Input: part model. Units: mm. Frame: model coordinates. Face numbers are marked on the shaded views. A direction names the side the tool comes from. Round coordinates to 2 decimals unless told otherwise and drop trailing zeros. Order: outer loops, then holes, each group sorted by start corner. A loop starts at its lowest first (then second) coordinate and runs counter-clockwise, first axis right, second up. Notation, with made-up numbers: M 5,-6 L 50,-6 A5 cw 50,2 Z; hole C 1,52 d2. An arc over 180 degrees is marked long. One line per question, with ' | ' between items.
Autodesk Inventor part; units mm, degrees
ref_plane "YZ Plane" through (0, 0, 0) normal (1, 0, 0) x (0, 1, 0)
ref_plane "XZ Plane" through (0, 0, 0) normal (0, 1, 0) x (-1, 0, 0)
ref_plane "XY Plane" through (0, 0, 0) normal (0, 0, 1) x (1, 0, 0)
sketch "Эскиз1" plane through (0, 0, 0) normal (0, 1, 0) x (-1, 0, 0)
  line L0 (54, 15) -> (-54, 15)
  line L1 (-54, 15) -> (-54, -15)
  line L2 (-54, -15) -> (54, -15)
  line L3 (54, -15) -> (54, 15)
  line L4 (-54, 15) -> (54, -15) construction
  line L5 (-54, -15) -> (54, 15) construction
  line L6 (0, -21) -> (0, 21) construction
  line L7 (44, -13) -> (7.0585, -13)
  line L8 (-44, -13) -> (-44, 13)
  line L9 (-44, 13) -> (0, 13)
  line L10 (44, 13) -> (44, 2.0855)
  line L11 (75.6, 0) -> (-75.6, 0) construction
  line L12 (49, -15) -> (49, 15) construction
  line L13 (0, -13) -> (44, 0)
  line L14 (44, -2.0855) -> (7.0585, -13)
  line L15 (0, -15) -> (0, -13) construction
  line L16 (0, 13) -> (0, 15) construction
  line L17 (44, -2.0855) -> (43.4333, -0.1674) construction
  line L18 (44, 0) -> (0, 13)
  line L19 (44, 2.0855) -> (7.0585, 13)
  line L20 (44, 2.0855) -> (43.4333, 0.1674) construction
  line L21 (44, 2.0855) -> (44, -2.0855) construction
  line L22 (44, -2.0855) -> (44, -13)
  line L23 (7.0585, -13) -> (0, -13) construction
  line L24 (0, -13) -> (-44, -13)
  line L25 (7.0585, 13) -> (44, 13)
  line L26 (0, 13) -> (7.0585, 13) construction
  point P0 (0, 0)
  point P1 (0, -14)
  point P2 (0, 14)
  point P3 (0, 0)
  dimension "d0" = 108
  dimension "d8" = 10
  dimension "d9" = 5
  dimension "d28" = 26
  dimension "d46" = 2
  dimension "d47" = 10
extrude "Выдавливание1" add sketch "Эскиз1" along normal blind 2
sketch "Эскиз2" plane through (0, 0, 0) normal (0, 1, 0) x (-1, 0, 0)
  line L0 (-42, -13) -> (-42, 13) construction
  line L1 (-42, -13) -> (-29, -13) construction
  line L2 (-10.5, -13) -> (-10.5, -15)
  line L3 (-10.5, -15) -> (-44, -15)
  line L4 (-42, 13) -> (-29, 13) construction
  line L5 (-10.5, 15) -> (-44, 15)
  line L6 (-10.5, 13) -> (-10.5, 15)
  arc A0 (-29, 13) -> (-29, -13) centre (-29, 0) ccw
  line L7 (-29, -13) -> (-10.5, -13)
  line L8 (-29, 13) -> (-10.5, 13)
  line L9 (-44, -15) -> (-44, 15)
  line L10 (-44, -13) -> (-44, 13) construction
  line L11 (0, -13) -> (-44, -13) construction
  line L12 (-54, -15) -> (54, -15) construction
  line L13 (-44, 13) -> (0, 13) construction
  line L14 (54, 15) -> (-54, 15) construction
  point P0 (0, 0)
  dimension "d17" = 31.5
  dimension "d48" = 2
extrude "Выдавливание2" add sketch "Эскиз2" along normal blind 13
sketch "Эскиз4" plane through (0, 2, 0) normal (0, 1, 0) x (1, 0, 0)
  line L0 (-54, 15) -> (-54, -15) construction
  line L1 (-44, 13) -> (-54, 13)
  line L2 (-54, 13) -> (-54, 15)
  line L3 (-54, 15) -> (-44, 15)
  line L4 (-44, 15) -> (-44, 13)
  line L5 (44, -13) -> (0, -13) construction
  line L6 (-54, -15) -> (54, -15) construction
  line L7 (-44, -13) -> (-54, -13)
  line L8 (-54, -13) -> (-54, -15)
  line L9 (-54, -15) -> (-44, -15)
  line L10 (-44, -15) -> (-44, -13)
  point P0 (0, 0)
  point P1 (10.5, -13)
  point P2 (-44, -15)
extrude "Выдавливание4" add sketch "Эскиз4" along normal blind 45
sketch "Эскиз3" plane through (-54, 0, 15) normal (0, 0, 1) x (1, 0, 0)
  line L0 (64.5, 2) -> (64.5, 13) construction
  line L1 (64.5, 13) -> (74.5, 13) construction
  line L2 (74.5, 13) -> (74.5, 3) construction
  line L3 (74.5, 3) -> (64.5, 3) construction
  line L4 (64.5, 3) -> (64.5, 13) construction
  line L5 (64.5, 2) -> (54, 2) construction
  line L6 (74.5, 3) -> (64.5, 13) construction
  line L7 (74.5, 13) -> (64.5, 3) construction
  circle A0 centre (69.5, 8) radius 0.5
  line L8 (0, 47) -> (10, 47) construction
  line L9 (10, 2) -> (10, 47) construction
  line L10 (0, 47) -> (10, 47) construction
  line L11 (10, 47) -> (10, 37) construction
  line L12 (10, 37) -> (0, 37) construction
  line L13 (0, 37) -> (0, 47) construction
  line L14 (0, 37) -> (10, 47) construction
  line L15 (0, 0) -> (0, 47) construction
  line L16 (10, 37) -> (0, 47) construction
  circle A1 centre (5, 42) radius 0.5
  point P0 (54, 0)
  point P1 (128, 2)
  dimension "d20" = 10
  dimension "d21" = 1
  dimension "d26" = 10
  dimension "d27" = 1
hole "Отверстие1" at (-49, 42, 15) at (15.5, 8, 15) direction (0, 0, -1) diameter 1 depth 2 countersink diameter 1.5 countersink angle 90
mirror "Зеркальное отражение1" about plane through (0, 0, 0) normal (0, 0, 1) of "Отверстие1"
sketch "Эскиз5" plane through (0, 2, 0) normal (0, 1, 0) x (1, 0, 0)
  line L0 (10.5, 13) -> (10.5, 15) construction
  line L1 (-44, 15) -> (10.5, 15) construction
  line L2 (-54, 15) -> (-44, 15) construction
  line L3 (-54, 13) -> (-54, 15) construction
  line L4 (-44, 13) -> (-54, 13) construction
  line L5 (-44, -13) -> (-44, -15) construction
  line L6 (-44, -15) -> (-54, -15) construction
  line L7 (-54, -15) -> (-54, -13) construction
  line L8 (-54, -13) -> (-54, 13) construction
  line L9 (10.5, -15) -> (10.5, -13) construction
  line L10 (10.5, 15) -> (44, 15) construction
  line L11 (54, -15) -> (44, -15) construction
  line L12 (54, 15) -> (54, -15) construction
  line L13 (44, 15) -> (54, 15) construction
  line L14 (-44, 15) -> (-44, 13) construction
  line L15 (-54, -13) -> (-44, -13) construction
  line L16 (44, -15) -> (10.5, -15) construction
  line L17 (54, 15) -> (-54, 15) construction
  line L18 (54, 15) -> (44, 0) construction
  line L19 (-54, -15) -> (54, -15) construction
  line L20 (54, -15) -> (44, 0) construction
  line L21 (-54, 13) -> (-44, -13) construction
  line L22 (-44, -13) -> (-44, -2.0855) construction
  line L23 (-54, -13) -> (-44, 13) construction
  line L24 (54, -15) -> (54, 15) construction
  line L25 (54, 0) -> (44, 15) construction
  line L26 (44, -15) -> (54, 0) construction
  circle A0 centre (-49, 0) radius 0.5
  circle A1 centre (49, 7.5) radius 0.5
  circle A2 centre (49, -7.5) radius 0.5
  line L27 (-44, 2.0855) -> (-7.0585, 13)
  line L28 (-7.0585, 13) -> (-44, 13)
  line L29 (-44, -13) -> (-7.0585, -13)
  line L30 (-7.0585, -13) -> (-44, -2.0855)
  line L31 (-44, -2.0855) -> (-44, -13)
  line L32 (-44, 13) -> (-44, 2.0855)
  line L33 (10.5, 13) -> (0, 13)
  line L34 (0, 13) -> (-44, 0)
  line L35 (-44, 0) -> (0, -13)
  line L36 (0, -13) -> (10.5, -13)
  line L37 (10.5, -13) -> (29, -13)
  arc A3 (29, -13) -> (29, 13) centre (29, 0) ccw
  line L38 (29, 13) -> (10.5, 13)
  line L39 (44, 15) -> (44, -15)
  line L40 (10.5, -15) -> (-44, -15)
  point P0 (0, 0)
  dimension "d38" = 1
hole "Отверстие2" at (-49, 2, 0) at (49, 2, 7.5) at (49, 2, -7.5) direction (0, -1, 0) diameter 1 end through all countersink diameter 1.5 countersink angle 90
properties part number "frame"
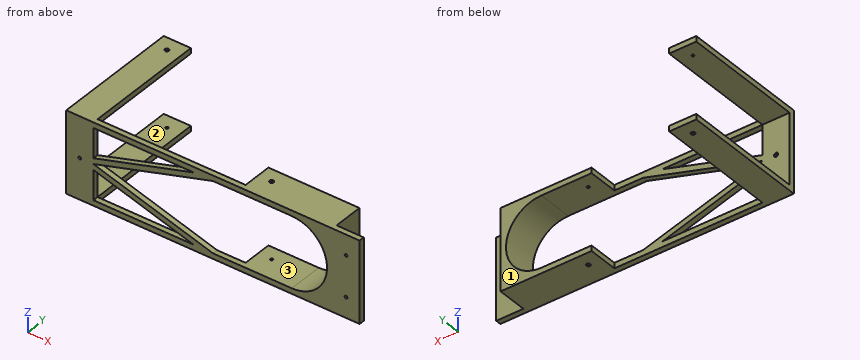
Item 1: Section query A-A, the plane y = 5.5. Return loops of the section in (x, z).
Report:
outline: M -54,-15 L -44,-15 L -44,-13 L -54,-13 Z; M -54,13 L -44,13 L -44,15 L -54,15 Z; M 10.5,-15 L 44,-15 L 44,15 L 10.5,15 L 10.5,13 L 29,13 A13 cw 29,-13 L 10.5,-13 Z
Item 2: Section query C-C, the plane y = 21.5. Return loops of the section in (x, z).
Report:
outline: M -54,-15 L -44,-15 L -44,-13 L -54,-13 Z; M -54,13 L -44,13 L -44,15 L -54,15 Z
Item 3: First-contact query: pin 1 (1 mm diameter, centred on y = 16, z = -14, fed in from +X); pin 2 (5 mm diameter, centred on y = 10, z = 0, fed in from +X); pin 3 (10 mm diameter, centred on x = -6.5, z = 6.5, fed in from +Y). Flat tips, straight axial feed; report the tip coordinate or a pass-through.
Report:
pin 1: x = -44 | pin 2: x = 44 | pin 3: y = 2
Item 4: Section query B-B, the plane x = 26.5. Return loops of the section in (y, z).
Report:
outline: M 0,-15 L 13,-15 L 13,-13 L 0,-13 Z; M 0,13 L 13,13 L 13,15 L 0,15 Z
Item 5: Line query: line 1 along X through (y, z) = (8, 14); line 2 along Y through (x, z) = (-49, -14.25); line 3 along Y through (x, z) = (15.5, 13.6). Output: solid intervals per line, ascending. Write a range as from..to.
Report:
line 1: -54..-44, 10.5..15, 16..44 | line 2: 0..41.5, 42.5..47 | line 3: 0..7.5, 8.5..13
Item 6: Section query D-D, the plane z = -9.5. Return loops of the section in (x, y), plus the area to 3 significant figures.
Report:
outline: M -54,0 L -44,0 L -44,2 L -54,2 Z; M -18.9,0 L -11.85,0 L -11.85,2 L -18.9,2 Z; M 37.87,0 L 54,0 L 54,2 L 44,2 L 44,13 L 37.87,13 Z | area: 134 mm²
Item 7: Access query for the marked faces 1, 2 and 3. Directions: +Z, -Z, +X, -X, +Y, -Y. A direction counts if a zero-diameter tool reaches every point of the face in a straight line with its end or side. Return the directions, or none.
Report:
face 1: +Z, -Z, +X, +Y | face 2: -X, +Y | face 3: +Y, -Y
